from build123d import *

# Parameters (mm, degrees)
EXTRUDE_1_DEPTH = 10
EXTRUDE_START   = -1.5
EXTRUDE_2_DEPTH = 8.5


with BuildPart() as part:
    # Эскиз1 → Бобышка-Вытянуть1 (new body)
    with BuildSketch(Plane.XY):
        with BuildLine():
            Line((-35, 22.2), (35, 22.2))
            ThreePointArc((35, 22.2), (40.091168825, 20.091168825), (42.2, 15))
            Line((42.2, 15), (42.2, -15))
            ThreePointArc((42.2, -15), (40.091168825, -20.091168825), (35, -22.2))
            Line((35, -22.2), (-35, -22.2))
            ThreePointArc((-35, -22.2), (-40.091168825, -20.091168825), (-42.2, -15))
            Line((-42.2, -15), (-42.2, 15))
            ThreePointArc((-42.2, 15), (-40.091168825, 20.091168825), (-35, 22.2))
        make_face()
        with BuildLine():
            Line((-40.2, -15), (-40.2, 15))
            ThreePointArc((-40.2, 15), (-38.676955262, 18.676955262), (-35, 20.2))
            Line((-35, 20.2), (35, 20.2))
            ThreePointArc((35, 20.2), (38.676955262, 18.676955262), (40.2, 15))
            Line((40.2, 15), (40.2, -15))
            ThreePointArc((40.2, -15), (38.676955262, -18.676955262), (35, -20.2))
            Line((35, -20.2), (-35, -20.2))
            ThreePointArc((-35, -20.2), (-38.676955262, -18.676955262), (-40.2, -15))
        make_face(mode=Mode.SUBTRACT)
    extrude(amount=EXTRUDE_1_DEPTH)

    # Эскиз2 → Бобышка-Вытянуть2 (add)
    with BuildSketch(Plane(origin=(0, 0, 0), x_dir=(-1, 0, 0), z_dir=(0, 0, -1)).offset(EXTRUDE_START)):
        with BuildLine():
            Line((31, 15), (31, 20.2))
            Line((31, 20.2), (35, 20.2))
            ThreePointArc((35, 20.2), (38.676955262, 18.676955262), (40.2, 15))
            Line((40.2, 15), (40.2, 11))
            Line((40.2, 11), (35, 11))
            ThreePointArc((35, 11), (32.171572875, 12.171572875), (31, 15))
        make_face()
        with BuildLine():
            Line((-35, 20.2), (-31, 20.2))
            Line((-31, 20.2), (-31, 15))
            ThreePointArc((-31, 15), (-32.171572875, 12.171572875), (-35, 11))
            Line((-35, 11), (-40.2, 11))
            Line((-40.2, 11), (-40.2, 15))
            ThreePointArc((-40.2, 15), (-38.676955262, 18.676955262), (-35, 20.2))
        make_face()
        with BuildLine():
            Line((-31, -15), (-31, -20.2))
            Line((-31, -20.2), (-35, -20.2))
            ThreePointArc((-35, -20.2), (-38.676955262, -18.676955262), (-40.2, -15))
            Line((-40.2, -15), (-40.2, -11))
            Line((-40.2, -11), (-35, -11))
            ThreePointArc((-35, -11), (-32.171572875, -12.171572875), (-31, -15))
        make_face()
        with BuildLine():
            Line((35, -20.2), (31, -20.2))
            Line((31, -20.2), (31, -15))
            ThreePointArc((31, -15), (32.171572875, -12.171572875), (35, -11))
            Line((35, -11), (40.2, -11))
            Line((40.2, -11), (40.2, -15))
            ThreePointArc((40.2, -15), (38.676955262, -18.676955262), (35, -20.2))
        make_face()
    extrude(amount=-EXTRUDE_2_DEPTH)


solid = part.part
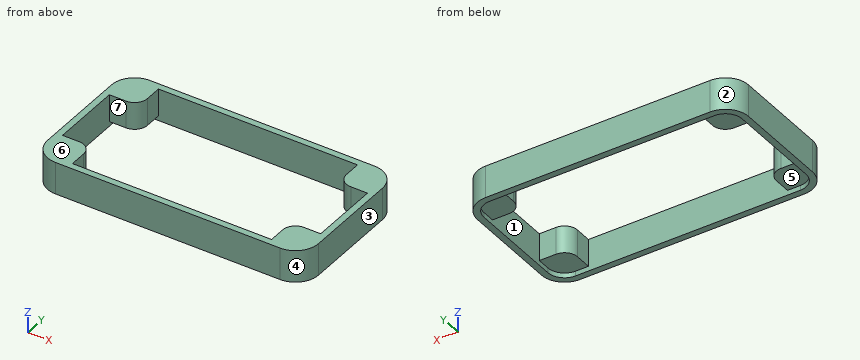
Geometry: final body of the model. Coordinates: model frame, mm. Face numbers are marked on the shaded views. A direction names the side the tool comes from. Coordinates: 2 decimals unless noted, no trailing zeros. Order: outer loops, then holes, each group sorted by start corner. A loop starts at its lowest first (then second) coordinate and runs counter-clockwise, first axis right, second up.
(1) Material intervals for probe 1 along Y at (x, z) = (-30.5, 8.75); probe 2 along X at (y, z) = (-2.5, 6.5); probe 3 along Z at (x, y) = (31.5, -14), sorted ascending.
(2) Draft query along Y for the marked faces 1, 2, 3 and 4. Return one class per face: pulls with the +Y half, pulls with the -Y half, needs draft (parallel to the pull), parting line crosses it, or undercut.
(3) Section query B-B (z = 4). Return the cut outline in (x, y), plus the area to 3 significant figures.
(4) First-contact query: pin 1 (3 mm diameter, centred on x = 36.5, y = -17, fed in from -Z); pin 2 (5.5 mm diameter, centred on y = 18.5, z = 7.5, fed in from +X); pin 3 (4 mm diameter, centred on y = -17.5, z = 4.5, fed in from -X). Flat tips, straight axial feed; report the tip coordinate or a pass-through.
(5) Section query D-D (y = -12.5). Return the cut outline in (x, z), plus the area to 3 significant figures.
(6) Section query C-C (y = 7.5). Return the cut outline in (x, z).
(7) Access query for the marked faces 5, 6 and 7. Directions: +Z, -Z, +X, -X, +Y, -Y. A direction counts if a zero-diameter tool reaches every point of the face in a straight line with its end or side. Return the directions, or none.
(8) Section query A-A (x = -7). Return the cut outline in (y, z).
Solution:
1. probe 1: y = -22.2 to -20.2, 20.2 to 22.2
1. probe 2: x = -42.2 to -40.2, 40.2 to 42.2
1. probe 3: z = 1.5 to 10
2. face 1: undercut
2. face 2: pulls with the +Y half
2. face 3: needs draft
2. face 4: pulls with the -Y half
3. outline: (-42.2, -15) arc R7.2 ccw to (-35, -22.2) - (35, -22.2) arc R7.2 ccw to (42.2, -15) - (42.2, 15) arc R7.2 ccw to (35, 22.2) - (-35, 22.2) arc R7.2 ccw to (-42.2, 15) - close; hole (-40.2, -11) - (-35, -11) arc R4 cw to (-31, -15) - (-31, -20.2) - (31, -20.2) - (31, -15) arc R4 cw to (35, -11) - (40.2, -11) - (40.2, 11) - (35, 11) arc R4 cw to (31, 15) - (31, 20.2) - (-31, 20.2) - (-31, 15) arc R4 cw to (-35, 11) - (-40.2, 11) - close
3. area: 780 mm2
4. pin 1: stops at z = 1.5
4. pin 2: stops at x = 42.16
4. pin 3: stops at x = -42.18
5. outline: (-42.2, 0) - (-40.2, 0) - (-40.2, 1.5) - (-31.88, 1.5) - (-31.88, 10) - (-42.2, 10) - close; (31.88, 1.5) - (40.2, 1.5) - (40.2, 0) - (42.2, 0) - (42.2, 10) - (31.88, 10) - close
5. area: 181 mm2
6. outline: (-42.2, 0) - (-40.2, 0) - (-40.2, 10) - (-42.2, 10) - close; (40.2, 0) - (42.2, 0) - (42.2, 10) - (40.2, 10) - close
7. face 5: -Z
7. face 6: +Z, +X, -X, +Y, -Y
7. face 7: +Z, -Z
8. outline: (-22.2, 0) - (-20.2, 0) - (-20.2, 10) - (-22.2, 10) - close; (20.2, 0) - (22.2, 0) - (22.2, 10) - (20.2, 10) - close
